For this review, take the finished solid that the model builds, in its own axes (mm). A direction names the side the tool comes from. Coordinates: 2 decimals unless noted, no trailing zeros. Write each loop counter-clockwise with the first axis right and the second up, starting at its lowest first coordinate (ties: lowest second). Pieces come first, ordered by that corner, then holes.
1) Insertion check: P1, Ø12, axis at x = 12.5, y = 21, coming from the +Z side; P2, Ø3, axis at y = -21.5, z = 7, coming from the +X side (3 decimals); P3, Ø9, axis at x = 74, y = 1.5, coming from the -Z side. Each pin has a flat end and moves straight along its axis. Give the tip position at first contact, or say it passes through.
2) We need section B-B on y = 29.5. Write out the cut boundary in (x, z) (3 decimals).
3) For faces 1 (the face through (21, 25.4, 36)), 2 (the face through (71, 0, 61.925)), 3 (the face through (1, -45, 9.525)), 4 (the face through (70, 0, 42.875)), list the 3-axis set-ups (+Z, -Z, +X, -X, +Y, -Y) from which the entire face can be reached by the end or side of a thin tool; tool diameter is ignored.
4) To check wall thickness, follow line 1 along X through (y, z) = (48.5, 8.5) (3 decimals); line 2 along Y through (x, z) = (1.5, 25); line 3 along Z through (x, y) = (36, 18) (3 decimals). State the ranges of each line that lie inside material, in increasing order.
5) We need section A-A on x = 73.5. Write out the cut boundary in (y, z).
from build123d import *

# Parameters (mm, degrees)
F1_DEPTH = 63.5
F0_W     = 25.196091
F0_H     = 19.05
F2_DEPTH = 25.4


with BuildPart() as f1:
    # F0 (on Front) → F1 (new body, symmetric)
    with BuildSketch(Plane.XZ):
        Polygon((22.225, 9.525), (-41.275, 9.525), (-41.275, -9.525), (41.275, -9.525), (41.275, 9.525), align=None)
    extrude(amount=F1_DEPTH, both=True)

    # F0 (on Front) → F2 (join, symmetric)
    with BuildSketch(Plane.XZ):
        with BuildLine():
            Line((22.225, 28.545261), (22.225, 9.525))
            Line((22.225, 9.525), (41.275, 9.525))
            Line((41.275, 9.525), (41.275, 28.545261))
            ThreePointArc((41.275, 28.545261), (45.472142, 38.678058), (55.604939, 42.8752))
            Line((55.604939, 42.8752), (60.528909, 42.8752))
            Line((60.528909, 42.8752), (60.528909, 61.9252))
            Line((60.528909, 61.9252), (55.604939, 61.9252))
            ThreePointArc((55.604939, 61.9252), (32.001758, 52.148442), (22.225, 28.545261))
        make_face()
        with Locations((73.126954, 52.4002)):
            Rectangle(F0_W, F0_H)
        with BuildLine():
            add(Edge.make_bspline(
                [(-41.275, 9.525), (-4.208209, 9.525), (-15.882595, 75.476266), (55.604939, 61.9252)],
                knots=[0, 0, 0, 0, 110.143105, 110.143105, 110.143105, 110.143105], degree=3))
            Line((-41.275, 9.525), (22.225, 9.525))
            Line((22.225, 9.525), (22.225, 28.545261))
            ThreePointArc((22.225, 28.545261), (32.001758, 52.148442), (55.604939, 61.9252))
        make_face()
    extrude(amount=F2_DEPTH, both=True)


solid = f1.part
Result:
1. P1: stops at z = 60.66
1. P2: stops at x = 41.275
1. P3: stops at z = 42.88
2. outline: (-41.275, -9.525) - (41.275, -9.525) - (41.275, 9.525) - (-41.275, 9.525) - close
3. face 1: +Z, +X, -X, +Y
3. face 2: +Z, +X, +Y, -Y
3. face 3: +Z, +X, -X, -Y
3. face 4: -Z, +X, +Y, -Y
4. line 1: x = -41.275 to 41.275
4. line 2: y = -25.4 to 25.4
4. line 3: z = -9.525 to 63.741
5. outline: (-25.4, 42.88) - (25.4, 42.88) - (25.4, 61.93) - (-25.4, 61.93) - close
